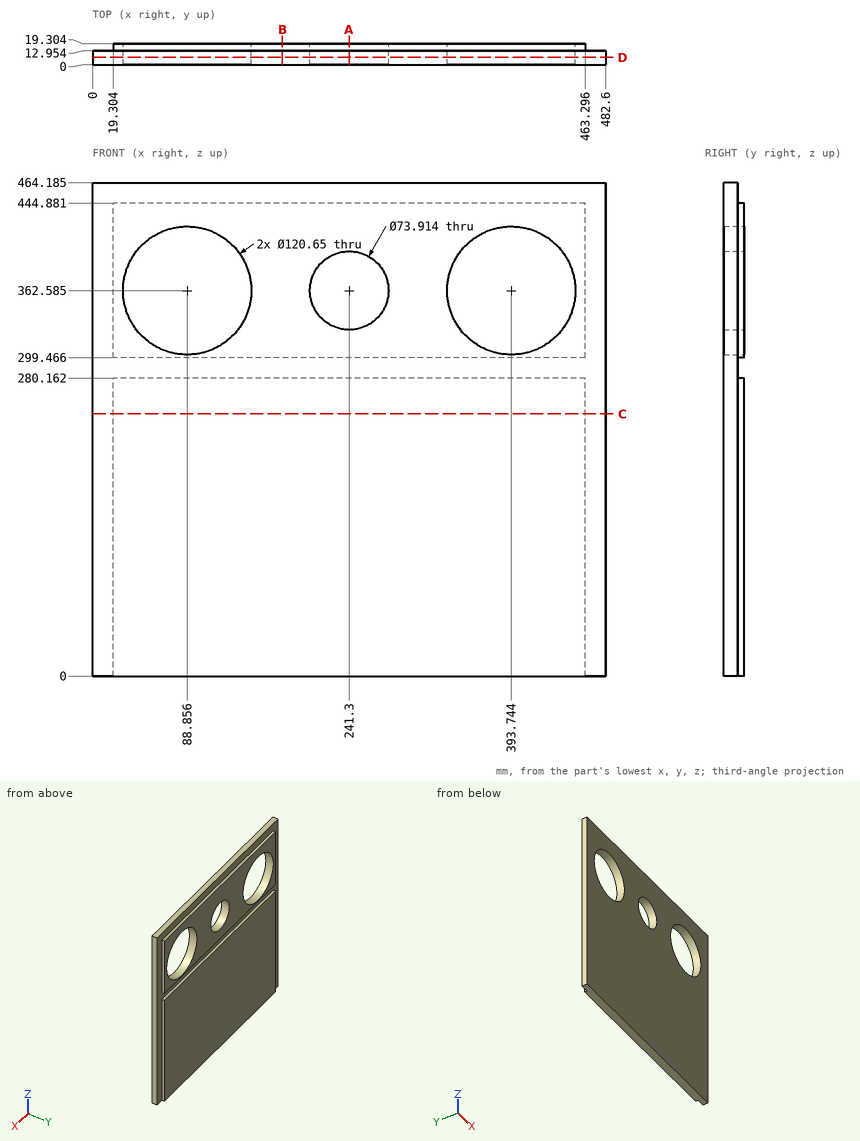
Print and shaded views of the part. All mm, measured from the part's lowest x, y and z. Give positions to 0.01 mm unless a question says otherwise; leave off trailing zeros. Loops run counter-clockwise (first coordinate to the right, second up) from the corner with the lowest first, then second, coordinate; pieces in that order, holes last.
1) Saw through at B-B (x = 178.5). Write the cut outline in (y, z) (1 decimal).
2) Saw through at A-A (x = 241.3). Write the cut outline in (y, z) (1 decimal).
3) Flat gauge pins, fed straight in: pin 1 Ø3 at (x, y) = (356, 15) entering from +Z; pin 2 Ø3 at (y, z) = (15, 370.5) entering from -X; pin 3 Ø1.9 at (y, z) = (17, 195) entering from +X. Where does each tip first touch, or does it go through?
4) Saw through at C-C (z = 246.5). Write the cut outline in (x, y).
5) Wall check: line 1 (Z direction, x = 103, y = 16.25) (1 decimal); line 2 (Z direction, x = 91.5, y = 6.75) (1 decimal); line 3 (Z direction, x = 96.5, y = 17.5) (1 decimal). Give the ranges that are in metal, low to high.
6) Saw through at D-D (y = 6.75). Count the separate pieces of the cut face and the enclosed holes in it, plus the area to 3 significant figures.
Answer block:
1. outline: (0, 0) - (19.3, 0) - (19.3, 280.2) - (13, 280.2) - (13, 299.5) - (19.3, 299.5) - (19.3, 444.9) - (13, 444.9) - (13, 464.2) - (0, 464.2) - close
2. outline: (0, 0) - (19.3, 0) - (19.3, 280.2) - (13, 280.2) - (13, 299.5) - (19.3, 299.5) - (19.3, 325.6) - (0, 325.6) - close; (0, 399.5) - (19.3, 399.5) - (19.3, 444.9) - (13, 444.9) - (13, 464.2) - (0, 464.2) - close
3. pin 1: stops at z = 444.88
3. pin 2: stops at x = 19.3
3. pin 3: stops at x = 463.3
4. outline: (0, 0) - (482.6, 0) - (482.6, 12.95) - (463.3, 12.95) - (463.3, 19.3) - (19.3, 19.3) - (19.3, 12.95) - (0, 12.95) - close
5. line 1: z = 0 to 280.2, 299.5 to 303.9, 421.2 to 444.9
5. line 2: z = 0 to 302.3, 422.9 to 464.2
5. line 3: z = 0 to 280.2, 299.5 to 302.7, 422.4 to 444.9
6. separate pieces: 1
6. enclosed holes: 3
6. area: 197,000 mm2
